Work out the finished part from the listing and answer in its coordinate system (mm). A direction names the side the tool comes from. Round coordinates to 2 decimals unless told otherwise and drop trailing zeros. Loops run counter-clockwise (first coordinate to the right, second up) from the corner with the lowest first, then second, coordinate; pieces in that order, holes last. Notation, with made-up numbers: (-21, 79.5) - (8, 79.5) arc R23 cw to (8, 107.5) - close; hole circle Ø1 at (26, 11). An arc over 180 degrees is marked (long way). Return JSON: item names as keys, results as strings.
from build123d import *

# Parameters (mm, degrees)
SKETCH_1_R      = 29.5
SKETCH_1_R_2    = 1.82136949
EXTRUDE_1_DEPTH = 10
SKETCH_2_R      = 5
EXTRUDE_2_DEPTH = 10


with BuildPart() as part:
    # 草图1 → 凸台-拉伸1 (new body)
    with BuildSketch(Plane.XY):
        Circle(SKETCH_1_R)
        with Locations((0, 17.25)):
            Circle(SKETCH_1_R_2, mode=Mode.SUBTRACT)
        with Locations((14.938938215, 8.625)):
            Circle(SKETCH_1_R_2, mode=Mode.SUBTRACT)
        with Locations((14.938938215, -8.625)):
            Circle(SKETCH_1_R_2, mode=Mode.SUBTRACT)
        with Locations((0, -17.25)):
            Circle(SKETCH_1_R_2, mode=Mode.SUBTRACT)
        with Locations((-14.938938215, -8.625)):
            Circle(SKETCH_1_R_2, mode=Mode.SUBTRACT)
        with Locations((-14.938938215, 8.625)):
            Circle(SKETCH_1_R_2, mode=Mode.SUBTRACT)
    extrude(amount=EXTRUDE_1_DEPTH)

    # 草图2 → 凸台-拉伸2 (add)
    with BuildSketch(Plane.XY.offset(10)):
        with Locations((-14.938938215, 8.625)):
            Circle(SKETCH_2_R)
    extrude(amount=EXTRUDE_2_DEPTH)


solid = part.part
1) Section C-C (x = -16) is taken. Give the vertices of the cut face in (y, z), and give its area (3 significant figures).
Verdict:
{"outline": "(-24.78, 0) - (-10.11, 0) - (-10.11, 10) - (-24.78, 10) - close; (-7.14, 0) - (7.14, 0) - (7.14, 10) - (10.11, 10) - (10.11, 0) - (24.78, 0) - (24.78, 10) - (13.51, 10) - (13.51, 20) - (3.74, 20) - (3.74, 10) - (-7.14, 10) - close", "area": "534 mm2"}
2) Section D-D (z = 8) is taken. Give the vertices of the cut face in (x, y) (3 decimals), and give its area (3 significant figures).
Verdict:
{"outline": "circle Ø59 at (0, 0); hole circle Ø3.643 at (-14.939, -8.625); hole circle Ø3.643 at (-14.939, 8.625); hole circle Ø3.643 at (0, -17.25); hole circle Ø3.643 at (0, 17.25); hole circle Ø3.643 at (14.939, -8.625); hole circle Ø3.643 at (14.939, 8.625)", "area": "2,670 mm2"}
3) Determine the mould class of faces 4 (the cylindrical face through (-13.2, -8.08, 4.93)), 5 (the flat face through (-15, 9, 20)), 6 (the cylindrical face through (28.14, 8.86, 4.93)) for opening direction Y: pulls with the +Y half, pulls with the -Y half, needs draft (parallel to the pull), parting line crosses it, or undercut.
Verdict:
{"face 4": "undercut", "face 5": "needs draft", "face 6": "parting line crosses it"}
4) A tool of negligible diameter and unlimited length cuts with its end or side. For faces 1 (the cylindrical face through (-13.2, 9.17, 4.93)), 2 (the cylindrical face through (-18.624, 12.004, 14.93)), 3 (the cylindrical face through (16.676, 9.172, 4.93)), from which of +Z, -Z, +X, -X, +Y, -Y can it reach the whole face along a straight path? Write none if from no direction.
Verdict:
{"face 1": "-Z", "face 2": "+Z", "face 3": "+Z, -Z"}
5) Section A-A (x = 0) is taken. Give the vertices of the cut face in (y, z), and give its area (3 significant figures).
Verdict:
{"outline": "(-29.5, 0) - (-19.07, 0) - (-19.07, 10) - (-29.5, 10) - close; (-15.43, 0) - (15.43, 0) - (15.43, 10) - (-15.43, 10) - close; (19.07, 0) - (29.5, 0) - (29.5, 10) - (19.07, 10) - close", "area": "517 mm2"}
6) Flat-ended cylindrical pins translate along their axes: pin 1 (6 mm diameter, centred on x = 14.94, y = -8.62, fed in from +Z); pin 2 (4 mm diameter, centred on x = 16, z = 8.5, fed in from -Y); pin 3 (1.5 mm diameter, centred on y = 13, z = 9, fed in from +X). Find the tip coordinate at first contact, or state that the pin passes through.
Verdict:
{"pin 1": "stops at z = 10", "pin 2": "stops at y = -25.97", "pin 3": "stops at x = 26.84"}
7) Section B-B (y = -17.25) is taken. Give the vertices of the cut face in (x, z).
Verdict:
{"outline": "(-23.93, 0) - (-1.82, 0) - (-1.82, 10) - (-23.93, 10) - close; (1.82, 0) - (23.93, 0) - (23.93, 10) - (1.82, 10) - close"}
8) Find the intervals of material crossed by L1, parallel to Y at x = 0, z = 2; L2, parallel to X at y = -9, z = 9; L3, parallel to Y at x = -13.5, z = 1.25, in increasing order.
Verdict:
{"L1": "y = -29.5 to -19.07, -15.43 to 15.43, 19.07 to 29.5", "L2": "x = -28.09 to -16.72, -13.16 to 13.16, 16.72 to 28.09", "L3": "y = -26.23 to -9.74, -7.51 to 7.51, 9.74 to 26.23"}
